```python
from build123d import *

# Parameters (mm, degrees)
SKETCH1_W           = 300
SKETCH1_H           = 300
SKETCH1_R           = 4
SKETCH1_W_2         = 15
SKETCH1_H_2         = 4
BOSS_EXTRUDE1_DEPTH = 4


with BuildPart() as part:
    # Sketch1 → Boss-Extrude1 (new body)
    with BuildSketch(Plane(origin=(0, 0, 0), x_dir=(1, 0, 0), z_dir=(0, 1, 0))):
        with Locations((-1.47665027, -0.17639355)):
            Rectangle(SKETCH1_W, SKETCH1_H)
        with Locations((-1e-09, 3e-09)):
            Circle(SKETCH1_R, mode=Mode.SUBTRACT)
        with Locations((44.999999999, 3e-09)):
            Circle(SKETCH1_R, mode=Mode.SUBTRACT)
        with Locations((22.499999999, 38.971143173)):
            Circle(SKETCH1_R, mode=Mode.SUBTRACT)
        with Locations((-22.500000001, 38.971143173)):
            Circle(SKETCH1_R, mode=Mode.SUBTRACT)
        with Locations((-45.000000001, 3e-09)):
            Circle(SKETCH1_R, mode=Mode.SUBTRACT)
        with Locations((-22.500000001, -38.971143168)):
            Circle(SKETCH1_R, mode=Mode.SUBTRACT)
        with Locations((22.499999999, -38.971143168)):
            Circle(SKETCH1_R, mode=Mode.SUBTRACT)
        with Locations((-71.47665027, 66.82360645)):
            Rectangle(SKETCH1_W_2, SKETCH1_H_2, mode=Mode.SUBTRACT)
        with Locations((-36.47665027, 66.82360645)):
            Rectangle(SKETCH1_W_2, SKETCH1_H_2, mode=Mode.SUBTRACT)
        with Locations((-1.47665027, 66.82360645)):
            Rectangle(SKETCH1_W_2, SKETCH1_H_2, mode=Mode.SUBTRACT)
        with Locations((33.52334973, 66.82360645)):
            Rectangle(SKETCH1_W_2, SKETCH1_H_2, mode=Mode.SUBTRACT)
        with Locations((68.52334973, 66.82360645)):
            Rectangle(SKETCH1_W_2, SKETCH1_H_2, mode=Mode.SUBTRACT)
        with Locations((68.52334973, -67.17639355)):
            Rectangle(SKETCH1_W_2, SKETCH1_H_2, mode=Mode.SUBTRACT)
        with Locations((33.52334973, -67.17639355)):
            Rectangle(SKETCH1_W_2, SKETCH1_H_2, mode=Mode.SUBTRACT)
        with Locations((-1.47665027, -67.17639355)):
            Rectangle(SKETCH1_W_2, SKETCH1_H_2, mode=Mode.SUBTRACT)
        with Locations((-36.47665027, -67.17639355)):
            Rectangle(SKETCH1_W_2, SKETCH1_H_2, mode=Mode.SUBTRACT)
        with Locations((-71.47665027, -67.17639355)):
            Rectangle(SKETCH1_W_2, SKETCH1_H_2, mode=Mode.SUBTRACT)
    extrude(amount=BOSS_EXTRUDE1_DEPTH)


solid = part.part
```
The model under review builds one solid part; all positions refer to its coordinate system, in mm. Coordinates: 2 decimals unless noted, no trailing zeros. Order: outer loops, then holes, each group sorted by start corner. A loop starts at its lowest first (then second) coordinate and runs counter-clockwise, first axis right, second up. Notation, with made-up numbers: (20.5, 57) -> (32.5, 57) arc R19 ccw to (32.5, 75) -> close; hole circle Ø6 at (-30, 6.5). An arc over 180 degrees is marked (long way). Answer in a Markdown table with one row per item. Add a question column.
Item 1: Mouldability with a two-part tool opening along X and no side actions: class faces 1 (the cylindrical face through (-0.867, 1.972, 3.905)), 2 (the flat face through (-4, 4, -2)) as +X half, -X half, draft (parallel to the pull), parting line (faces both ways), or undercut.
Item 2: To check wall thickness, follow probe 1 along Z at (x, y) = (22.5, 2.55); probe 2 along X at (y, z) = (2.5, 0); probe 3 along Z at (x, y) = (72.5, 1.65). State the ranges of each line that lie inside material, in increasing order.
Item 3: We need section B-B on x = -22.5. Write out the cut boundary in (y, z).
Item 4: We need section A-A on z = 0. Write out the cut boundary in (x, y), plus the area to 3 significant figures.
Item 5: We need section C-C on x = 45. Write out the cut boundary in (y, z), plus the area to 3 significant figures.
Final values:
| question | item | result |
|---|---|---|
| 1 | face 1 | undercut |
| 1 | face 2 | draft |
| 2 | probe 1 | z = -149.82 to -42.97, -34.97 to 34.97, 42.97 to 150.18 |
| 2 | probe 2 | x = -151.48 to -49, -41 to -4, 4 to 41, 49 to 148.52 |
| 2 | probe 3 | z = -149.82 to -68.82, -64.82 to 65.18, 69.18 to 150.18 |
| 3 | outline | (0, -149.82) -> (4, -149.82) -> (4, -42.97) -> (0, -42.97) -> close; (0, -34.97) -> (4, -34.97) -> (4, 34.97) -> (0, 34.97) -> close; (0, 42.97) -> (4, 42.97) -> (4, 150.18) -> (0, 150.18) -> close |
| 4 | outline | (-151.48, 0) -> (-49, 0) -> (-49, 4) -> (-151.48, 4) -> close; (-41, 0) -> (-4, 0) -> (-4, 4) -> (-41, 4) -> close; (4, 0) -> (41, 0) -> (41, 4) -> (4, 4) -> close; (49, 0) -> (148.52, 0) -> (148.52, 4) -> (49, 4) -> close |
| 4 | area | 1,100 mm2 |
| 5 | outline | (0, -149.82) -> (4, -149.82) -> (4, -4) -> (0, -4) -> close; (0, 4) -> (4, 4) -> (4, 150.18) -> (0, 150.18) -> close |
| 5 | area | 1,170 mm2 |
